Here's how the part is built. I have some questions about the finished solid (model axes, mm). Face numbers are marked on the shaded views. A direction names the side the tool comes from. Give positions to 0.01 mm unless a question says otherwise; leave off trailing zeros. Write each loop counter-clockwise with the first axis right and the second up, starting at its lowest first coordinate (ties: lowest second). Pieces come first, ordered by that corner, then holes. Notation, with made-up numbers: (-39.5, -11) -> (-29.5, -11) arc R35 cw to (-29.5, 22) -> close; hole circle Ø10 at (-15, 88). An arc over 180 degrees is marked (long way). Return JSON: item names as keys, results as strings.
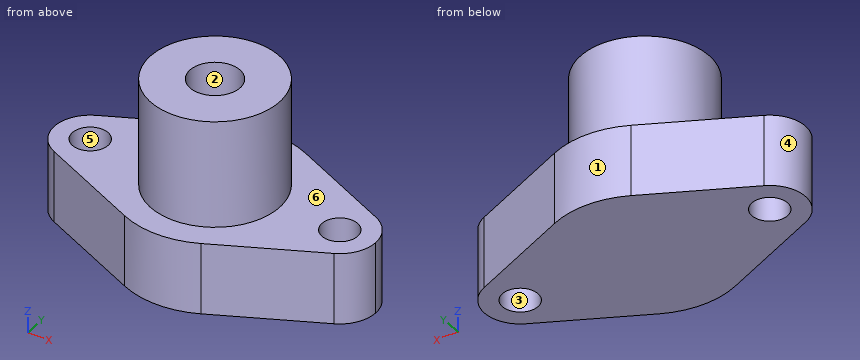
from build123d import *

# Parameters (mm, degrees)
F1_DEPTH = 20
F2_DEPTH = 30
F3_D     = 10
F5_D     = 14
F5_DEPTH = 31
F5_TIP   = 4.2060243332


with BuildPart() as f1:
    # F0 (on Top) → F1 (new body)
    with BuildSketch(Plane.XY):
        with BuildLine():
            Line((-39.2857142857, -9.0350790291), (-10.7142857143, -22.5876975726))
            ThreePointArc((-10.7142857143, -22.5876975726), (-21.1288563682, -13.3630620956), (-25, 0))
            ThreePointArc((-25, 0), (-29.6547751618, -8.4515425473), (-39.2857142857, -9.0350790291))
        make_face()
        with BuildLine():
            ThreePointArc((-39.2857142857, -9.0350790291), (-29.6547751618, -8.4515425473), (-25, 0))
            ThreePointArc((-25, 0), (-29.6547751618, 8.4515425473), (-39.2857142857, 9.0350790291))
            ThreePointArc((-39.2857142857, 9.0350790291), (-45, 0), (-39.2857142857, -9.0350790291))
        make_face()
        with BuildLine():
            Line((0, 0), (18, 0))
            ThreePointArc((18, 0), (0, 18), (-18, 0))
            Line((-18, 0), (0, 0))
        make_face()
        with BuildLine():
            ThreePointArc((-18, 0), (0, -18), (18, 0))
            Line((18, 0), (0, 0))
            Line((0, 0), (-18, 0))
        make_face()
        with BuildLine():
            ThreePointArc((10.7142857143, -22.5876975726), (21.1288563682, -13.3630620956), (25, 0))
            Line((25, 0), (18, 0))
            ThreePointArc((18, 0), (0, -18), (-18, 0))
            Line((-18, 0), (-25, 0))
            ThreePointArc((-25, 0), (-21.1288563682, -13.3630620956), (-10.7142857143, -22.5876975726))
            ThreePointArc((-10.7142857143, -22.5876975726), (0, -25), (10.7142857143, -22.5876975726))
        make_face()
        with BuildLine():
            ThreePointArc((39.2857142857, -9.0350790291), (29.6547751618, -8.4515425473), (25, 0))
            ThreePointArc((25, 0), (21.1288563682, -13.3630620956), (10.7142857143, -22.5876975726))
            Line((10.7142857143, -22.5876975726), (39.2857142857, -9.0350790291))
        make_face()
        with BuildLine():
            ThreePointArc((39.2857142857, 9.0350790291), (29.6547751618, 8.4515425473), (25, 0))
            ThreePointArc((25, 0), (29.6547751618, -8.4515425473), (39.2857142857, -9.0350790291))
            ThreePointArc((39.2857142857, -9.0350790291), (43.4515425473, -5.3452248382), (45, 0))
            ThreePointArc((45, 0), (43.4515425473, 5.3452248382), (39.2857142857, 9.0350790291))
        make_face()
        with BuildLine():
            ThreePointArc((10.7142857143, 22.5876975726), (21.1288563682, 13.3630620956), (25, 0))
            ThreePointArc((25, 0), (29.6547751618, 8.4515425473), (39.2857142857, 9.0350790291))
            Line((39.2857142857, 9.0350790291), (10.7142857143, 22.5876975726))
        make_face()
        with BuildLine():
            ThreePointArc((-25, 0), (-21.1288563682, 13.3630620956), (-10.7142857143, 22.5876975726))
            Line((-10.7142857143, 22.5876975726), (-39.2857142857, 9.0350790291))
            ThreePointArc((-39.2857142857, 9.0350790291), (-29.6547751618, 8.4515425473), (-25, 0))
        make_face()
        with BuildLine():
            Line((18, 0), (25, 0))
            ThreePointArc((25, 0), (21.1288563682, 13.3630620956), (10.7142857143, 22.5876975726))
            ThreePointArc((10.7142857143, 22.5876975726), (0, 25), (-10.7142857143, 22.5876975726))
            ThreePointArc((-10.7142857143, 22.5876975726), (-21.1288563682, 13.3630620956), (-25, 0))
            Line((-25, 0), (-18, 0))
            ThreePointArc((-18, 0), (0, 18), (18, 0))
        make_face()
    extrude(amount=-F1_DEPTH)

    # F0 (on Top) → F2 (join)
    with BuildSketch(Plane.XY):
        with BuildLine():
            Line((0, 0), (18, 0))
            ThreePointArc((18, 0), (0, 18), (-18, 0))
            Line((-18, 0), (0, 0))
        make_face()
        with BuildLine():
            ThreePointArc((-18, 0), (0, -18), (18, 0))
            Line((18, 0), (0, 0))
            Line((0, 0), (-18, 0))
        make_face()
    extrude(amount=F2_DEPTH)

    # F3 (through all)
    with Locations(Plane.XY):
        with Locations((-35, 0), (35, 0)):
            Hole(F3_D / 2)

    # F5
    with Locations(Plane.XY.offset(30)):
        with Locations((0, 0)):
            Hole(F5_D / 2, depth=F5_DEPTH)
            with Locations((0, 0, -(F5_DEPTH + F5_TIP / 2))):  # 118° drill point
                Cone(0, F5_D / 2, F5_TIP, mode=Mode.SUBTRACT)


solid = f1.part
1. Suppose I cut it at D-D, the plane z = 15. List the corners of the cut face in (x, y) for me.
Taken from the geometry:
{"outline": "circle Ø36 at (0, 0); hole circle Ø14 at (0, 0)"}
2. If I drill on line 1 (X direction, y = -1, z = -9); line 2 (Z direction, x = 38.5, y = -5); line 3 (X direction, y = 0, z = 19.5), over which ranges is the centre line in solid material (lowest first)? Write a range as [from, to].
Taken from the geometry:
{"line 1": "x = [-44.95, -39.9], [-30.1, 30.1], [39.9, 44.95]", "line 2": "z = [-20, 0]", "line 3": "x = [-18, -7], [7, 18]"}
3. Suppose I cut it at B-B, the plane x = 35. List the corners of the cut face in (y, z) for me.
Taken from the geometry:
{"outline": "(-11.07, -20) -> (-5, -20) -> (-5, 0) -> (-11.07, 0) -> close; (5, -20) -> (11.07, -20) -> (11.07, 0) -> (5, 0) -> close"}
4. For pin 1 Ø12 at (x, z) = (11.5, 7.5) entering from +Y; pin 2 Ø6 at (y, z) = (-14, 22.5) entering from +X; pin 3 Ø11 at (x, y) = (0, 0) entering from +Z, each with a flat end and sliding along its axis, tell me the tip position at first contact or that it passes through.
Taken from the geometry:
{"pin 1": "stops at y = 17.14", "pin 2": "stops at x = 14.25", "pin 3": "stops at z = -1.9"}
5. Suppose I cut it at C-C, the plane y = -14. List the corners of the cut face in (x, z) for me.
Taken from the geometry:
{"outline": "(-28.82, -20) -> (28.82, -20) -> (28.82, 0) -> (11.31, 0) -> (11.31, 30) -> (-11.31, 30) -> (-11.31, 0) -> (-28.82, 0) -> close"}
6. If we mould it in two halves opening along Y, with no side actions, what happens to the marked faces 3, 4, 5 and 6? For each: released by +Y, released by -Y, zero draft, split by the parting line, or undercut.
Taken from the geometry:
{"face 3": "undercut", "face 4": "split by the parting line", "face 5": "undercut", "face 6": "zero draft"}
7. Suppose I cut it at A-A, the plane z = -14. List the corners of the cut face in (x, y) for me.
Taken from the geometry:
{"outline": "(-39.29, -9.04) -> (-10.71, -22.59) arc R25 ccw to (10.71, -22.59) -> (39.29, -9.04) arc R10 ccw to (39.29, 9.04) -> (10.71, 22.59) arc R25 ccw to (-10.71, 22.59) -> (-39.29, 9.04) arc R10 ccw to start; hole circle Ø10 at (-35, 0); hole circle Ø10 at (35, 0)"}
8. Which directions (+Z, -Z, +X, -X, +Y, -Y) give clear straight access to the entire face, cutting with the end or side of a thin tool? Please do the marked faces 1 and 2.
Taken from the geometry:
{"face 1": "+Z, -Z, +Y", "face 2": "+Z"}
